Autodesk Inventor part; units mm, degrees
ref_plane "YZ Plane" through (0, 0, 0) normal (1, 0, 0) x (0, 1, 0)
ref_plane "XZ Plane" through (0, 0, 0) normal (0, 1, 0) x (-1, 0, 0)
ref_plane "XY Plane" through (0, 0, 0) normal (0, 0, 1) x (1, 0, 0)
sketch "Sketch1" plane through (0, 0, 0) normal (1, 0, 0) x (0, 1, 0)
  circle A0 centre (0, 0) radius 6
  dimension "d0" = 12
extrude "Extrusion1" add sketch "Sketch1" along normal blind 5
sketch "Sketch2" plane through (5, 0, 0) normal (1, 0, 0) x (0, 0, -1)
  circle A0 centre (0, 0) radius 6
  circle A1 centre (0, 0) radius 6.5
  dimension "d3" = 13
extrude "Extrusion2" add sketch "Sketch2" along normal blind 0.5 contours A0 | A1
chamfer "Chamfer1" distance 0.25 angle 45 1 edges at (5.5, 0, 6.5)
sketch "Sketch3" plane through (5.5, 0, 0) normal (1, 0, 0) x (0, 0, -1)
  circle A0 centre (0, 0) radius 6.25
  circle A1 centre (0, 0) radius 3
  dimension "d9" = 6
extrude "Extrusion3" cut sketch "Sketch3" against normal blind 5 contours A1
properties part number "500-138" material "ABS Plastic"
Input: part model. Units: mm. Frame: model coordinates. A direction names the side the tool comes from. Give positions to 0.01 mm unless a question says otherwise; leave off trailing zeros. Loops run counter-clockwise (first coordinate to the right, second up) from the corner with the lowest first, then second, coordinate; pieces in that order, holes last. Notation, with made-up numbers: (6, 87.25) - (40, 87.25) arc R21 ccw to (40, 98.25) - close; hole circle Ø8 at (41.25, -9). An arc over 180 degrees is marked (long way). Use CSV: the item, a comma, the result in double quotes. Start each with the question number.
Item 1: Line query: line 1 (X direction, y = -1.5, z = 1); line 2 (Y direction, x = 2.35, z = -2.25); line 3 (Z direction, x = 1.1, y = 2). Output: solid intervals per line, ascending.
Item 2: Contact query for flat-ended pins moving along their axis: P1, Ø7, axis at y = 0, z = 0, coming from the +X side; P2, Ø2, axis at x = 3.5, z = 0, coming from the +Y side; P3, Ø2, axis at y = -1.5, z = 0.5, coming from the +X side; P4, Ø1, axis at x = 1.5, y = -3.5, coming from the -Z side. Output: stop coordinate, or through.
Item 3: Section B-B on z = 0. Return loops of the section in (x, y), then the cut area to 3 significant figures.
Item 4: Mould query, pull axis Y, two halves, no side actions, for faces 1 (the cylindrical face through (2, -6, 0)), 2 (the flat face through (5.5, -3, 1)), 3 (the flat face through (0.5, 0, 0)). Classes: pulls with the +Y half, pulls with the -Y half, needs draft (parallel to the pull), parting line crosses it, or undercut.
Item 5: Reachability of faces 4 (the cylindrical face through (3, 0, 3)), 5 (the flat face through (0, 0, 0)), 6 (the flat face through (5, -6, -2)) from +Z, -Z, +X, -X, +Y, -Y: full face, straight path, thin tool, end or side. Return the list, or none.
Item 6: Section A-A on x = 1.9. Return loops of the section in (y, z).
Ans:
1,line 1,"x = 0 to 0.5"
1,line 2,"y = -5.56 to -1.98, 1.98 to 5.56"
1,line 3,"z = -5.66 to -2.24, 2.24 to 5.66"
2,P1,"stops at x = 5.5"
2,P2,"stops at y = 6"
2,P3,"stops at x = 0.5"
2,P4,"stops at z = -5.2"
3,outline,"(0, -6) - (5, -6) - (5, -6.5) - (5.25, -6.5) - (5.5, -6.25) - (5.5, -3) - (0.5, -3) - (0.5, 3) - (5.5, 3) - (5.5, 6.25) - (5.25, 6.5) - (5, 6.5) - (5, 6) - (0, 6) - close"
3,area,"36.4 mm2"
4,face 1,"parting line crosses it"
4,face 2,"needs draft"
4,face 3,"undercut"
5,face 4,"+X"
5,face 5,"+Z, -Z, -X, +Y, -Y"
5,face 6,"-X"
6,outline,"circle Ø12 at (0, 0); hole circle Ø6 at (0, 0)"
